Build history of the part. All positions in model axes, mm. A direction names the side the tool comes from. Coordinates: 2 decimals unless noted, no trailing zeros. Order: outer loops, then holes, each group sorted by start corner. A loop starts at its lowest first (then second) coordinate and runs counter-clockwise, first axis right, second up. Notation, with made-up numbers: (37.5, 48) - (44.5, 48) arc R21 ccw to (44.5, 53) - close; hole circle Ø7 at (-4, 13.25). An arc over 180 degrees is marked (long way). One line per item, written item: value.
Autodesk Inventor part; units mm, degrees
ref_plane "YZ Plane" through (0, 0, 0) normal (1, 0, 0) x (0, 1, 0)
ref_plane "XZ Plane" through (0, 0, 0) normal (0, 1, 0) x (-1, 0, 0)
ref_plane "XY Plane" through (0, 0, 0) normal (0, 0, 1) x (1, 0, 0)
sketch "Sketch1" plane through (0, 0, 0) normal (0, 0, 1) x (1, 0, 0)
  line L0 (-7.1784, -0.1841) -> (0.0716, -0.1841)
  line L1 (0.0716, -0.1841) -> (0.0716, -7.4341)
  line L2 (0.0716, -7.4341) -> (-7.1784, -7.4341)
  line L3 (-7.1784, -7.4341) -> (-7.1784, -0.1841)
  line L4 (-7.1784, -2.1841) -> (-5.1784, -2.1841)
  line L5 (-5.1784, -2.1841) -> (-5.1784, -0.1841)
  line L6 (-1.9284, -0.1841) -> (-1.9284, -2.1841)
  line L7 (-1.9284, -2.1841) -> (0.0716, -2.1841)
  line L8 (-7.1784, -5.4341) -> (-5.1784, -5.4341)
  line L9 (-5.1784, -5.4341) -> (-5.1784, -7.4341)
  line L10 (-1.9284, -5.4341) -> (0.0716, -5.4341)
  line L11 (-1.9284, -5.4341) -> (-1.9284, -7.4341)
  line L12 (8.0716, 0.8159) -> (8.0716, -8.4341)
  line L13 (-15.1784, -8.4341) -> (-15.1784, 0.8159)
  circle A0 centre (-12.1784, -3.8091) radius 1.25
  circle A1 centre (5.0716, -3.8091) radius 1.25
  line L14 (-15.1784, 0.8159) -> (-9.1784, 0.8159)
  line L15 (-9.1784, 0.8159) -> (-9.1784, -8.4341)
  line L16 (-9.1784, -8.4341) -> (-15.1784, -8.4341)
  line L17 (-15.1784, -8.4341) -> (-15.1784, 0.8159)
  line L18 (8.0716, 0.8159) -> (2.0716, 0.8159)
  line L19 (2.0716, 0.8159) -> (2.0716, -8.4341)
  line L20 (2.0716, -8.4341) -> (8.0716, -8.4341)
  line L21 (8.0716, -8.4341) -> (8.0716, 0.8159)
  line L22 (-9.1784, 0.8159) -> (2.0716, 0.8159)
  line L23 (-9.1784, -8.4341) -> (2.0716, -8.4341)
  line L24 (-15.1784, 0.8159) -> (-21.6784, 0.8159)
  line L25 (-21.6784, 0.8159) -> (-21.6784, -8.4341)
  line L26 (-21.6784, -8.4341) -> (-15.1784, -8.4341)
  line L27 (-15.1784, -8.4341) -> (-15.1784, 0.8159)
  circle A2 centre (-18.4284, -3.8091) radius 2.625
  point P0 (0, 0)
  dimension "d0" = 7.25
  dimension "d1" = 7.25
  dimension "d2" = 2
  dimension "d3" = 2
  dimension "d4" = 2
  dimension "d5" = 2
  dimension "d6" = 8
  dimension "d7" = 8
  dimension "d10" = 2.5
  dimension "d11" = 2.5
  dimension "d12" = 6
  dimension "d13" = 6
  dimension "d14" = 3
  dimension "d15" = 3
  dimension "d23" = 1
  dimension "d24" = 1
  dimension "d25" = 9.25
  dimension "d26" = 4.625
  dimension "d27" = 4.625
  dimension "d28" = 17.25
  dimension "d29" = 5.25
  dimension "d30" = 3.25
  dimension "d31" = 6.5
  dimension "d33" = 6.25
extrude "Extrusion1" add sketch "Sketch1" along normal blind 1.5 contours L0 L6 L7 L1 L10 L11 L2 L9 L8 L3 L4 L5 | L12 L20 L19 L18 | L19 L23 L15 L22 | L15 L16 L13 L14
extrude "Extrusion2" add sketch "Sketch1" against normal blind 3.5 contours L12 L20 L19 L18 | L19 L23 L15 L22 | L15 L16 L13 L14
extrude "Extrusion3" add sketch "Sketch1" against normal blind 6.5 contours L12 L20 L19 L18 | L15 L16 L13 L14
equation "\"d2\" = d5"
equation "\"d3\" = d5"
equation "\"d4\" = d5"
equation "\"d13\" = d12"
equation "\"d15\" = d14"
equation "\"d26\" = 0.5 * d25"
equation "\"d27\" = d26"
properties part number "tac switch body"
1. Flat gauge pins, fed straight in: P1, Ø3.5, axis at x = -2.5, y = -2, coming from the -Z side; P2, Ø3, axis at x = -2, y = -7.5, coming from the -Z side. Where does each tip first touch, or does it go through?
Values found:
P1: stops at z = 0
P2: stops at z = -3.5
2. Two-plate mould, pull along Y, no slides. Class faces 1 (the face through (-4, -8.434, -2)), 2 (the face through (-15.178, -4, -3)), 3 (the face through (-1.928, -1, 1)): pulls with the +Y half, pulls with the -Y half, needs draft (parallel to the pull), parting line crosses it, or undercut.
Values found:
face 1: pulls with the -Y half
face 2: needs draft
face 3: undercut
3. Band-saw the part on A-A, the plane x = -1. Give the cut face in (y, z).
Values found:
outline: (-8.43, -3.5) - (-7.43, -3.5) - (-7.43, 1.5) - (-8.43, 1.5) - close; (-5.43, 0) - (-2.18, 0) - (-2.18, 1.5) - (-5.43, 1.5) - close; (-0.18, -3.5) - (0.82, -3.5) - (0.82, 1.5) - (-0.18, 1.5) - close
4. Probe line 1 along X through (y, z) = (-5.25, -6); line 2 along X through (y, z) = (-2.25, -2.75); line 3 along Y through (x, z) = (-3, -2.75). List the from-to ranges inside material, lowest first.
Values found:
line 1: x = -15.18 to -9.18, 2.07 to 8.07
line 2: x = -15.18 to -7.18, 0.07 to 8.07
line 3: y = -8.43 to -7.43, -0.18 to 0.82
5. 3-axis set-ups, long thin cutter, end or side, ignore diameter. For faces 4 (the face through (2.072, -4, -5)), 5 (the face through (3.7, -2.7, -6.5)), 6 (the face through (-1.928, -6, 1)), 7 (the face through (-7.178, -4, -2)), 8 (the face through (-4, -4, 1.5)): which of +Z, -Z, +X, -X, +Y, -Y reach the whole face in a straight line?
Values found:
face 4: -Z, +Y, -Y
face 5: -Z, +X, -X, +Y, -Y
face 6: +Z, -Z
face 7: -Z
face 8: +Z, +X, -X, +Y, -Y
6. Band-saw the part on D-D, the plane x = -4. Give the cut face in (y, z), and give its area (3 significant figures).
Values found:
outline: (-8.43, -3.5) - (-7.43, -3.5) - (-7.43, 0) - (-0.18, 0) - (-0.18, -3.5) - (0.82, -3.5) - (0.82, 1.5) - (-8.43, 1.5) - close
area: 20.9 mm2
7. Band-saw the part on B-B, the plane z = -4. Give the cut face in (x, y).
Values found:
outline: (-15.18, -8.43) - (-9.18, -8.43) - (-9.18, 0.82) - (-15.18, 0.82) - close; (2.07, -8.43) - (8.07, -8.43) - (8.07, 0.82) - (2.07, 0.82) - close; hole circle Ø2.5 at (-12.18, -3.81); hole circle Ø2.5 at (5.07, -3.81)
8. Band-saw the part on C-C, the plane y = -6. Give the cut face in (x, z).
Values found:
outline: (-15.18, -6.5) - (-9.18, -6.5) - (-9.18, -3.5) - (-7.18, -3.5) - (-7.18, 1.5) - (-15.18, 1.5) - close; (-5.18, 0) - (-1.93, 0) - (-1.93, 1.5) - (-5.18, 1.5) - close; (0.07, -3.5) - (2.07, -3.5) - (2.07, -6.5) - (8.07, -6.5) - (8.07, 1.5) - (0.07, 1.5) - close
